For this review, take the finished solid that the model builds, in its own axes (mm). Coordinates: 2 decimals unless noted, no trailing zeros. Loops run counter-clockwise (first coordinate to the right, second up) from the corner with the lowest first, then second, coordinate; pieces in that order, holes last. Notation, with made-up numbers: M 60,-16 L 98,-16 A21 cw 98,0 Z; hole C 8,56 d11. An arc over 180 degrees is marked long. Write item = value, one per line.
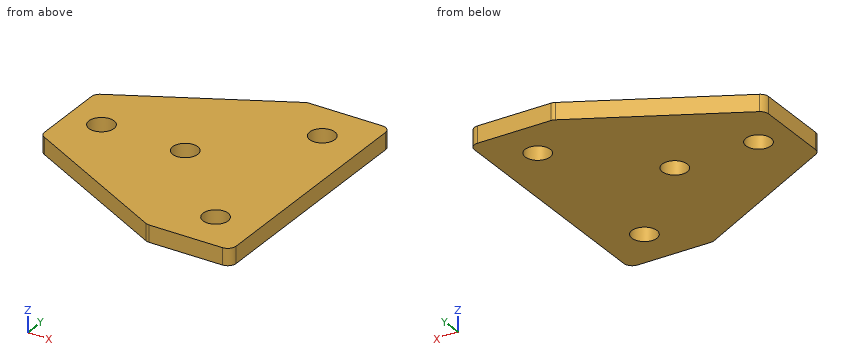
from build123d import *

# Parameters (mm, degrees)
SKETCH_1_R      = 1.5
EXTRUDE_1_DEPTH = 2
FILLET_1_R      = 1


with BuildPart() as part:
    # 草图1 → 凸台-拉伸1 (new body)
    with BuildSketch(Plane.XY):
        Polygon((0, 15), (0, -15), (-10, -15), (-29, -5), (-29, 5), (-10, 15), align=None)
        with Locations((-15, 0)):
            Circle(SKETCH_1_R, mode=Mode.SUBTRACT)
        with Locations((-5, -10)):
            Circle(SKETCH_1_R, mode=Mode.SUBTRACT)
        with Locations((-5, 10)):
            Circle(SKETCH_1_R, mode=Mode.SUBTRACT)
        with Locations((-25, 0)):
            Circle(SKETCH_1_R, mode=Mode.SUBTRACT)
    extrude(amount=EXTRUDE_1_DEPTH)

    # 圆角1
    fillet_1_edges = [part.edges().sort_by_distance(p)[0] for p in [
        (0, 15, 1),
        (0, -15, 1),
        (-10, -15, 1),
        (-29, -5, 1),
        (-29, 5, 1),
        (-10, 15, 1),
    ]]
    fillet(fillet_1_edges, radius=FILLET_1_R)


solid = part.part
Q1. Add section C-C (y = -10). Write out the cut boundary in (x, z).
Solved:
outline = M -19.5,0 L -6.5,0 L -6.5,2 L -19.5,2 Z; M -3.5,0 L 0,0 L 0,2 L -3.5,2 Z
Q2. Add section A-A (z = 0.5). Write out the cut boundary in (x, y), and give its area (3 significant figures).
Solved:
outline = M -29,-4.4 A1 ccw -28.47,-5.28 L -10.22,-14.88 A1 ccw -9.75,-15 L -1,-15 A1 ccw 0,-14 L 0,14 A1 ccw -1,15 L -9.75,15 A1 ccw -10.22,14.88 L -28.47,5.28 A1 ccw -29,4.4 Z; hole C -25,0 d3; hole C -15,0 d3; hole C -5,-10 d3; hole C -5,10 d3
area = 651 mm²
Q3. Add section D-D (x = -15). Write out the cut boundary in (y, z), and give its area (3 significant figures).
Solved:
outline = M -12.37,0 L -1.5,0 L -1.5,2 L -12.37,2 Z; M 1.5,0 L 12.37,0 L 12.37,2 L 1.5,2 Z
area = 43.5 mm²
Q4. For line 1 along Y through (x, z) = (-5, 1.15); line 2 along X through (y, z) = (0.75, 1.15); line 3 along X through (y, z) = (-4.5, 1.1), list the stretches that pass through material, from the lowest coordinate up.
Solved:
line_1 = -15 to -11.5, -8.5 to 8.5, 11.5 to 15
line_2 = -29 to -26.3, -23.7 to -16.3, -13.7 to 0
line_3 = -28.99 to 0
Q5. Add section B-B (y = 0). Write out the cut boundary in (x, z).
Solved:
outline = M -29,0 L -26.5,0 L -26.5,2 L -29,2 Z; M -23.5,0 L -16.5,0 L -16.5,2 L -23.5,2 Z; M -13.5,0 L 0,0 L 0,2 L -13.5,2 Z
